```python
from build123d import *

# Parameters (mm, degrees)
SKETCH1_R           = 6.25
BOSS_EXTRUDE1_DEPTH = 14
SKETCH2_R           = 2.1
CUT_EXTRUDE1_DEPTH  = 12
CUT_EXTRUDE2_DEPTH  = 7


with BuildPart() as part:
    # Sketch1 → Boss-Extrude1 (new body)
    with BuildSketch(Plane(origin=(0, 0, 0), x_dir=(1, 0, 0), z_dir=(0, 1, 0))):
        Circle(SKETCH1_R)
    extrude(amount=BOSS_EXTRUDE1_DEPTH)

    # Sketch2 → Cut-Extrude1 (cut)
    with BuildSketch(Plane(origin=(0, 14, 0), x_dir=(1, 0, 0), z_dir=(0, 1, 0))):
        Circle(SKETCH2_R)
    extrude(amount=-CUT_EXTRUDE1_DEPTH, mode=Mode.SUBTRACT)

    # Sketch3 → Cut-Extrude2 (cut, symmetric)
    with BuildSketch(Plane(origin=(0, 0, 0), x_dir=(0, 0, -1), z_dir=(1, 0, 0))):
        Polygon((2.25, 14), (6.25, 10), (6.25, 14), align=None)
    extrude(amount=CUT_EXTRUDE2_DEPTH, both=True, mode=Mode.SUBTRACT)


solid = part.part
```
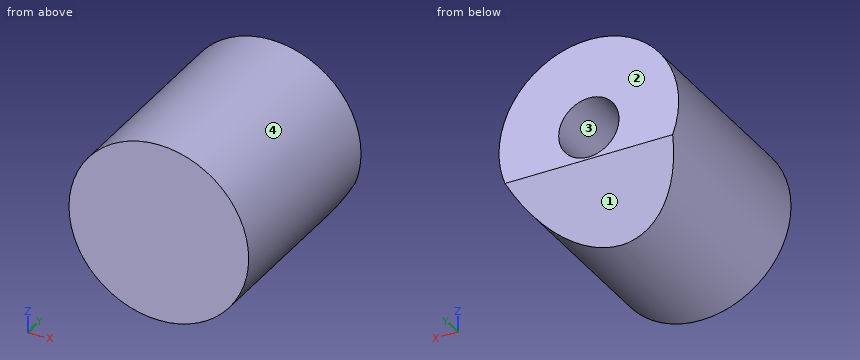
Check sheet for the modelled part. Datum: model origin and axes. Units: mm. Face numbers are marked on the shaded views. Give positions to 0.01 mm unless a question says otherwise; leave off trailing zeros. Write each loop counter-clockwise with the first axis right and the second up, starting at its lowest first coordinate (ties: lowest second). Pieces come first, ordered by that corner, then holes.
Item 1: Gauge pin test, flat ends, axial feed: pin 1 (6 mm diameter, centred on y = 12.5, z = -4, fed in from -X); pin 2 (6 mm diameter, centred on x = 4.5, y = 12, fed in from +Z). Record the tip position at first contact, or that the pin passes through.
Item 2: Cross-section at D-D (z = 5). Enter the section's corners in (x, y).
Item 3: Cross-section at C-C (y = 3.75). Enter the section's corners in (x, z).
Item 4: Cross-section at A-A (x = 0). Enter the section's corners in (y, z), and give its area (3 significant figures).
Item 5: Draft check along Z on the marked faces 1, 2, 3 and 4. Enter one of: released by +Z, released by -Z, zero draft, split by the parting line, or undercut.
Item 6: Scan lines: L1, parallel to X at y = 6.25, z = 0; L2, parallel to Z at x = -1, y = 12. Record each from-to range of solid material in increasing order.
Item 7: Cross-section at B-B (z = 0). Enter the section's corners in (x, y), and give its area (3 significant figures).
Report:
1. pin 1: stops at x = -6.17
1. pin 2: stops at z = 6.07
2. outline: (-3.75, 0) - (3.75, 0) - (3.75, 14) - (-3.75, 14) - close
3. outline: circle Ø12.5 at (0, 0); hole circle Ø4.2 at (0, 0)
4. outline: (0, -6.25) - (10, -6.25) - (14, -2.25) - (14, -2.1) - (2, -2.1) - (2, 2.1) - (14, 2.1) - (14, 6.25) - (0, 6.25) - close
4. area: 117 mm2
5. face 1: released by -Z
5. face 2: zero draft
5. face 3: undercut
5. face 4: split by the parting line
6. L1: x = -6.25 to -2.1, 2.1 to 6.25
6. L2: z = -4.25 to -1.85, 1.85 to 6.17
7. outline: (-6.25, 0) - (6.25, 0) - (6.25, 14) - (2.1, 14) - (2.1, 2) - (-2.1, 2) - (-2.1, 14) - (-6.25, 14) - close
7. area: 125 mm2
